from build123d import *

# Parameters (mm, degrees)
SKETCH1_R           = 18
SKETCH1_R_2         = 2
SKETCH1_W           = 10.25
SKETCH1_H           = 10.25
BOSS_EXTRUDE1_DEPTH = 36
CUT_EXTRUDE1_START  = -7
CUT_EXTRUDE1_DEPTH  = 7
SKETCH4_W           = 9.35
SKETCH4_H           = 9.35
CUT_EXTRUDE3_DEPTH  = 20.4
CUT_EXTRUDE4_START  = -40
CUT_EXTRUDE4_DEPTH  = 40
SKETCH6_R           = 1.5
CUT_EXTRUDE5_DEPTH  = 53.687759489
SKETCH7_R           = 3
CUT_EXTRUDE6_DEPTH  = 3
CUT_EXTRUDE7_DEPTH  = 4
CHAMFER1_SIZE       = 1
CHAMFER1_SIZE_2     = 2.747477419
CUT_EXTRUDE8_DEPTH  = 44.69210455
SKETCH12_R          = 1.4
CUT_EXTRUDE10_DEPTH = 20
SKETCH13_R          = 20
SKETCH13_R_2        = 1.4
BOSS_EXTRUDE2_DEPTH = 3
BOSS_EXTRUDE3_DEPTH = 3


with BuildPart() as part:
    # Sketch1 → Boss-Extrude1 (new body)
    with BuildSketch(Plane(origin=(0, 0, 0), x_dir=(1, 0, 0), z_dir=(0, 1, 0))):
        with Locations(Location((0, 0, 0), (0, 0, 270))):
            Circle(SKETCH1_R)
        with Locations(Location((-12, 0, 0), (0, 0, 270))):
            Circle(SKETCH1_R_2, mode=Mode.SUBTRACT)
        Rectangle(SKETCH1_W, SKETCH1_H, mode=Mode.SUBTRACT)
    extrude(amount=BOSS_EXTRUDE1_DEPTH)

    # Sketch2 → Cut-Extrude1 (cut)
    with BuildSketch(Plane(origin=(0, 36, 0), x_dir=(1, 0, 0), z_dir=(0, 1, 0)).offset(CUT_EXTRUDE1_START)):
        with BuildLine():
            Line((-10.8, 5), (-17.291616466, 5))
            ThreePointArc((-17.291616466, 5), (-18, 0), (-17.291616466, -5))
            Line((-17.291616466, -5), (-10.8, -5))
            ThreePointArc((-10.8, -5), (-5.8, 0), (-10.8, 5))
        make_face()
    extrude(amount=CUT_EXTRUDE1_DEPTH, mode=Mode.SUBTRACT)

    # Sketch4 → Cut-Extrude3 (cut)
    with BuildSketch(Plane(origin=(0, 0, 0), x_dir=(-1, 0, 0), z_dir=(0, -1, 0))):
        with Locations((11.135393506, 0.872889968)):
            Rectangle(SKETCH4_W, SKETCH4_H)
    extrude(amount=-CUT_EXTRUDE3_DEPTH, mode=Mode.SUBTRACT)

    # Sketch5 → Cut-Extrude4 (cut)
    with BuildSketch(Plane(origin=(0, 36, 0), x_dir=(1, 0, 0), z_dir=(0, 1, 0)).offset(CUT_EXTRUDE4_START)):
        with BuildLine():
            Line((5.916079783, 17), (-5.916079783, 17))
            ThreePointArc((-5.916079783, 17), (0, 18), (5.916079783, 17))
        make_face()
        with BuildLine():
            Line((5.916079783, -17), (-5.916079783, -17))
            ThreePointArc((-5.916079783, -17), (0, -18), (5.916079783, -17))
        make_face()
    extrude(amount=CUT_EXTRUDE4_DEPTH, mode=Mode.SUBTRACT)

    # Sketch6 → Cut-Extrude5 (cut, through all)
    with BuildSketch(Plane(origin=(0, 0, -17), x_dir=(-1, 0, 0), z_dir=(0, 0, -1))):
        with Locations((0, 26)):
            Circle(SKETCH6_R)
        with Locations((0, 5)):
            Circle(SKETCH6_R)
    extrude(amount=-CUT_EXTRUDE5_DEPTH, mode=Mode.SUBTRACT)

    # Sketch7 → Cut-Extrude6 (cut)
    with BuildSketch(Plane(origin=(0, 0, -17), x_dir=(-1, 0, 0), z_dir=(0, 0, -1))):
        with Locations((0, 26)):
            Circle(SKETCH7_R)
        with Locations((0, 5)):
            Circle(SKETCH7_R)
    extrude(amount=-CUT_EXTRUDE6_DEPTH, mode=Mode.SUBTRACT)

    # Sketch8 → Cut-Extrude7 (cut)
    with BuildSketch(Plane.XY.offset(17)):
        Polygon((0, 22.8), (2.771281292, 24.4), (2.771281292, 27.6), (0, 29.2), (-2.771281292, 27.6), (-2.771281292, 24.4), align=None)
        Polygon((0, 1.8), (2.771281292, 3.4), (2.771281292, 6.6), (0, 8.2), (-2.771281292, 6.6), (-2.771281292, 3.4), align=None)
    extrude(amount=-CUT_EXTRUDE7_DEPTH, mode=Mode.SUBTRACT)

    # Chamfer1
    # the kernel refuses this chamfer: 2.747477419, 1 mm, written as the material it takes off along each edge
    with BuildSketch(Plane(origin=(-5.125, 36, -5.125), x_dir=(0, 0.09904090225204956, -0.9950833631817488), z_dir=(1, 0, 0)), Plane(origin=(-5.125, 36, 5.125), x_dir=(-0.9950833631817488, 0.09904090225204956, 0), z_dir=(0, 0, -1)), Plane(origin=(5.125, 36, 5.125), x_dir=(0, 0.09904090225204956, 0.9950833631817488), z_dir=(-1, 0, 0)), Plane(origin=(5.125, 36, -5.125), x_dir=(0.9950833631817488, 0.09904090225204956, 0), z_dir=(0, 0, 1))) as chamfer1_piece_1:
        Polygon((CHAMFER1_SIZE * 0.995083363182, -CHAMFER1_SIZE * 0.099040902252), (-CHAMFER1_SIZE_2 * 0.0990409022684, -CHAMFER1_SIZE_2 * 0.995083363346), (0, 0), align=None)
    extrude(amount=10.25, mode=Mode.SUBTRACT)
    with BuildSketch(Plane(origin=(-5.125, 36, 5.125), x_dir=(-0.9950833631817488, 0.09904090225204956, 0), z_dir=(0, 0, -1))) as chamfer1_piece_2a_section:
        Polygon((CHAMFER1_SIZE * 0.995083363182, -CHAMFER1_SIZE * 0.099040902252), (-CHAMFER1_SIZE_2 * 0.0990409022684, -CHAMFER1_SIZE_2 * 0.995083363346), (0, 0), align=None)
    chamfer1_piece_2a = extrude(amount=17.377491449, mode=Mode.PRIVATE)
    chamfer1_piece_2a = split(chamfer1_piece_2a, bisect_by=Plane(origin=(-5.432505006, 35.059901151, -5.125), z_dir=(0, 0, -1)), keep=Keep.TOP, mode=Mode.PRIVATE)
    with BuildSketch(Plane(origin=(-12.252491449, 36, -5.125), x_dir=(0, 0.09904090225204956, -0.9950833631817488), z_dir=(1, 0, 0))) as chamfer1_piece_2b_section:
        Polygon((CHAMFER1_SIZE * 0.995083363182, -CHAMFER1_SIZE * 0.099040902252), (-CHAMFER1_SIZE_2 * 0.0990409022684, -CHAMFER1_SIZE_2 * 0.995083363346), (0, 0), align=None)
    chamfer1_piece_2b = extrude(amount=17.377491449, mode=Mode.PRIVATE)
    chamfer1_piece_2b = split(chamfer1_piece_2b, bisect_by=Plane(origin=(-5.125, 35.059901151, -5.432505006), z_dir=(-1, 0, 0)), keep=Keep.TOP, mode=Mode.PRIVATE)
    chamfer1_piece_2 = chamfer1_piece_2a & chamfer1_piece_2b
    add(chamfer1_piece_2, mode=Mode.SUBTRACT)
    with BuildSketch(Plane(origin=(5.125, 36, -12.252491449), x_dir=(0.9950833631817488, 0.09904090225204956, 0), z_dir=(0, 0, 1))) as chamfer1_piece_3a_section:
        Polygon((CHAMFER1_SIZE * 0.995083363182, -CHAMFER1_SIZE * 0.099040902252), (-CHAMFER1_SIZE_2 * 0.0990409022684, -CHAMFER1_SIZE_2 * 0.995083363346), (0, 0), align=None)
    chamfer1_piece_3a = extrude(amount=17.377491449, mode=Mode.PRIVATE)
    chamfer1_piece_3a = split(chamfer1_piece_3a, bisect_by=Plane(origin=(5.432505006, 35.059901151, -5.125), z_dir=(0, 0, -1)), keep=Keep.TOP, mode=Mode.PRIVATE)
    with BuildSketch(Plane(origin=(-5.125, 36, -5.125), x_dir=(0, 0.09904090225204956, -0.9950833631817488), z_dir=(1, 0, 0))) as chamfer1_piece_3b_section:
        Polygon((CHAMFER1_SIZE * 0.995083363182, -CHAMFER1_SIZE * 0.099040902252), (-CHAMFER1_SIZE_2 * 0.0990409022684, -CHAMFER1_SIZE_2 * 0.995083363346), (0, 0), align=None)
    chamfer1_piece_3b = extrude(amount=17.377491449, mode=Mode.PRIVATE)
    chamfer1_piece_3b = split(chamfer1_piece_3b, bisect_by=Plane(origin=(5.125, 35.059901151, -5.432505006), z_dir=(1, 0, 0)), keep=Keep.TOP, mode=Mode.PRIVATE)
    chamfer1_piece_3 = chamfer1_piece_3a & chamfer1_piece_3b
    add(chamfer1_piece_3, mode=Mode.SUBTRACT)
    with BuildSketch(Plane(origin=(5.125, 36, 5.125), x_dir=(0, 0.09904090225204956, 0.9950833631817488), z_dir=(-1, 0, 0))) as chamfer1_piece_4a_section:
        Polygon((CHAMFER1_SIZE * 0.995083363182, -CHAMFER1_SIZE * 0.099040902252), (-CHAMFER1_SIZE_2 * 0.0990409022684, -CHAMFER1_SIZE_2 * 0.995083363346), (0, 0), align=None)
    chamfer1_piece_4a = extrude(amount=17.377491449, mode=Mode.PRIVATE)
    chamfer1_piece_4a = split(chamfer1_piece_4a, bisect_by=Plane(origin=(-5.125, 35.059901151, 5.432505006), z_dir=(-1, 0, 0)), keep=Keep.TOP, mode=Mode.PRIVATE)
    with BuildSketch(Plane(origin=(-5.125, 36, 12.252491449), x_dir=(-0.9950833631817488, 0.09904090225204956, 0), z_dir=(0, 0, -1))) as chamfer1_piece_4b_section:
        Polygon((CHAMFER1_SIZE * 0.995083363182, -CHAMFER1_SIZE * 0.099040902252), (-CHAMFER1_SIZE_2 * 0.0990409022684, -CHAMFER1_SIZE_2 * 0.995083363346), (0, 0), align=None)
    chamfer1_piece_4b = extrude(amount=17.377491449, mode=Mode.PRIVATE)
    chamfer1_piece_4b = split(chamfer1_piece_4b, bisect_by=Plane(origin=(-5.432505006, 35.059901151, 5.125), z_dir=(0, 0, 1)), keep=Keep.TOP, mode=Mode.PRIVATE)
    chamfer1_piece_4 = chamfer1_piece_4a & chamfer1_piece_4b
    add(chamfer1_piece_4, mode=Mode.SUBTRACT)
    with BuildSketch(Plane(origin=(12.252491449, 36, 5.125), x_dir=(0, 0.09904090225204956, 0.9950833631817488), z_dir=(-1, 0, 0))) as chamfer1_piece_5a_section:
        Polygon((CHAMFER1_SIZE * 0.995083363182, -CHAMFER1_SIZE * 0.099040902252), (-CHAMFER1_SIZE_2 * 0.0990409022684, -CHAMFER1_SIZE_2 * 0.995083363346), (0, 0), align=None)
    chamfer1_piece_5a = extrude(amount=17.377491449, mode=Mode.PRIVATE)
    chamfer1_piece_5a = split(chamfer1_piece_5a, bisect_by=Plane(origin=(5.125, 35.059901151, 5.432505006), z_dir=(1, 0, 0)), keep=Keep.TOP, mode=Mode.PRIVATE)
    with BuildSketch(Plane(origin=(5.125, 36, -5.125), x_dir=(0.9950833631817488, 0.09904090225204956, 0), z_dir=(0, 0, 1))) as chamfer1_piece_5b_section:
        Polygon((CHAMFER1_SIZE * 0.995083363182, -CHAMFER1_SIZE * 0.099040902252), (-CHAMFER1_SIZE_2 * 0.0990409022684, -CHAMFER1_SIZE_2 * 0.995083363346), (0, 0), align=None)
    chamfer1_piece_5b = extrude(amount=17.377491449, mode=Mode.PRIVATE)
    chamfer1_piece_5b = split(chamfer1_piece_5b, bisect_by=Plane(origin=(5.432505006, 35.059901151, 5.125), z_dir=(0, 0, 1)), keep=Keep.TOP, mode=Mode.PRIVATE)
    chamfer1_piece_5 = chamfer1_piece_5a & chamfer1_piece_5b
    add(chamfer1_piece_5, mode=Mode.SUBTRACT)

    # Sketch9 → Cut-Extrude8 (cut, through all)
    with BuildSketch(Plane.XZ):
        with BuildLine():
            Line((-7.454203172, -7.297889968), (-15.454203172, -7.297889968))
            ThreePointArc((-15.454203172, -7.297889968), (-13.761984914, -9.955415688), (-11.632322635, -12.277178848))
            Line((-11.632322635, -12.277178848), (-7.454203172, -7.297889968))
        make_face()
    extrude(amount=-CUT_EXTRUDE8_DEPTH, mode=Mode.SUBTRACT)

    # Sketch12 → Cut-Extrude10 (cut)
    with BuildSketch(Plane(origin=(0, 36, 0), x_dir=(1, 0, 0), z_dir=(0, 1, 0))):
        with Locations(Location((10, 0, 0), (0, 0, 270))):
            Circle(SKETCH12_R)
        with Locations(Location((-9.192388155, -9.192388155, 0), (0, 0, 270))):
            Circle(SKETCH12_R)
    extrude(amount=-CUT_EXTRUDE10_DEPTH, mode=Mode.SUBTRACT)

    # Sketch13 → Boss-Extrude2 (add)
    with BuildSketch(Plane(origin=(0, 36, 0), x_dir=(1, 0, 0), z_dir=(0, 1, 0))):
        with Locations(Location((0, 0, 0), (0, 0, 270))):
            Circle(SKETCH13_R)
        with Locations(Location((10, 0, 0), (0, 0, 270))):
            Circle(SKETCH13_R_2, mode=Mode.SUBTRACT)
        with Locations(Location((-9.192388155, -9.192388155, 0), (0, 0, 270))):
            Circle(SKETCH13_R_2, mode=Mode.SUBTRACT)
        with BuildLine():
            Line((-10.8, 5), (-17.291616466, 5))
            Line((-17.291616466, 5), (-17.291616466, -5))
            Line((-17.291616466, -5), (-10.8, -5))
            ThreePointArc((-10.8, -5), (-7.959770503, -4.114984375), (-6.125, -1.773238563))
            Line((-6.125, -1.773238563), (-6.125, -6.125))
            Line((-6.125, -6.125), (6.125, -6.125))
            Line((6.125, -6.125), (6.125, 6.125))
            Line((6.125, 6.125), (-6.125, 6.125))
            Line((-6.125, 6.125), (-6.125, 1.773238563))
            ThreePointArc((-6.125, 1.773238563), (-7.959770503, 4.114984375), (-10.8, 5))
        make_face(mode=Mode.SUBTRACT)
        with BuildLine():
            Line((-7.454203172, 7.297889968), (-15.454203172, 7.297889968))
            ThreePointArc((-15.454203172, 7.297889968), (-13.761984914, 9.955415688), (-11.632322635, 12.277178848))
            Line((-11.632322635, 12.277178848), (-7.454203172, 7.297889968))
        make_face(mode=Mode.SUBTRACT)
    extrude(amount=BOSS_EXTRUDE2_DEPTH)

    # Sketch14 → Boss-Extrude3 (add)
    with BuildSketch(Plane(origin=(0, 39, 0), x_dir=(1, 0, 0), z_dir=(0, 1, 0))):
        with BuildLine():
            Line((12.855752194, 15.320888862), (14.321646009, 13.960317173))
            ThreePointArc((14.321646009, 13.960317173), (14.268984946, 15.373549926), (12.855752194, 15.320888862))
        make_face()
    extrude(amount=-BOSS_EXTRUDE3_DEPTH)


solid = part.part
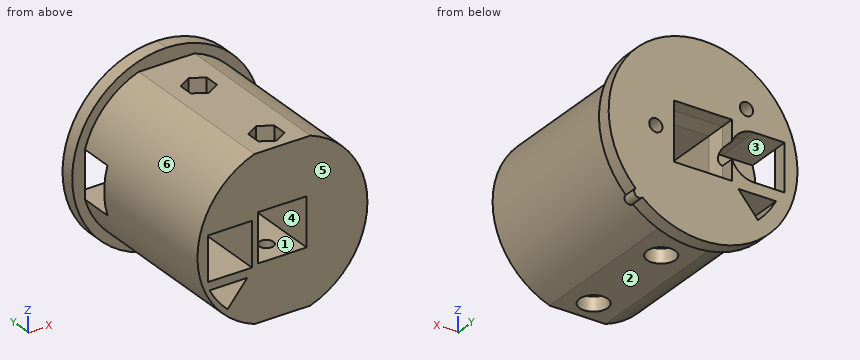
CAD build for the part. Positions are in the model's coordinates, mm. Face numbers are marked on the shaded views. A direction names the side the tool comes from. Coordinates: 2 decimals unless noted, no trailing zeros. Write each loop counter-clockwise with the first axis right and the second up, starting at its lowest first coordinate (ties: lowest second). Pieces come first, ordered by that corner, then holes. Notation, with made-up numbers: M 72.5,85.25 L 91.5,85.25 A12 ccw 91.5,96.25 Z; hole C 11.25,28.5 d7. An arc over 180 degrees is marked long. Answer as a JSON object with one key per item and string values. Group by question number.
1) Saw through at C-C (y = 19). Write the cut outline in (x, z) (3 decimals).
2) Saw through at D-D (z = -4). Write the cut outline in (x, y) (3 decimals), plus the area to 3 significant figures.
3) Mould opens along Z. For the marked faces 4, 5 and 6 say: +Z half, -Z half, draft (parallel to the pull), parting line (faces both ways), or undercut.
4) Saw through at A-A (y = 26). Give the number of separate pieces and of enclosed holes in the cut face, plus the area to 3 significant figures.
5) Saw through at B-B (z = -9.5). Write the cut outline in (x, y), plus the area to 3 significant figures.
6) Wall check: line 1 (X direction, y = 24.5, z = 0) (3 decimals); line 2 (Y direction, x = 0, z = -15); line 3 (Y direction, x = 0, z = -9). Give the ranges that are in metal, low to high. Write a range as from..to.
7) Pin check, flat tips, straight feed: pin 1 Ø5 at (x, y) = (-15, 32) entering from -Z; pin 2 Ø1.5 at (y, z) = (21, 14) entering from -X; pin 3 Ø8 at (y, z) = (14.5, -1) entering from +X. Stop position of each tip, or through.
8) Tool access for the marked faces 1, 2 and 3: list every direction of +Z, -Z, +X, -X, +Y, -Y with a clear straight run to the whole face (end or side of a thin tool).
Values follow:
{
 "1": {"outline": "M -5.916,-17 L 5.916,-17 A18 ccw 5.916,17 L -5.916,17 A18 ccw Z; hole M -15.81,-5.548 L -6.46,-5.548 L -6.46,3.802 L -15.81,3.802 Z; hole M -15.454,-7.298 A18 ccw -11.632,-12.277 L -7.454,-7.298 Z; hole C -9.192,9.192 d2.8; hole M -5.125,-5.125 L 5.125,-5.125 L 5.125,5.125 L -5.125,5.125 Z; hole C 10,0 d2.8"},
 "2": {"outline": "M -19.596,36 L -17.292,36 L -17.292,39 L -19.596,39 Z; M -17.55,0 L -15.81,0 L -15.81,20.4 L -6.46,20.4 L -6.46,0 L -5.125,0 L -5.125,33.253 L -6.125,36 L -6.125,39 L -7.8,39 L -7.8,29 L -17.55,29 Z; M 5.125,0 L 17.55,0 L 17.55,36 L 19.596,36 L 19.596,39 L 6.125,39 L 6.125,36 L 5.125,33.253 Z", "area": "685 mm2"},
 "3": {"face 4": "undercut", "face 5": "draft", "face 6": "parting line"},
 "4": {"separate pieces": "2", "enclosed holes": "4", "area": "761 mm2"},
 "5": {"outline": "M -17.6,36 L -15.29,36 L -15.29,0 L -14.1,0 L -14.1,39 L -17.6,39 Z; M -9.3,0 L 15.29,0 L 15.29,36 L 17.6,36 L 17.6,39 L -9.3,39 Z; hole C 0,5 d3; hole C 0,26 d3", "area": "1,010 mm2"},
 "6": {"line 1": "x = -18..-14, -10..-5.125, 5.125..8.6, 11.4..18", "line 2": "y = 0..2, 8..23, 29..39", "line 3": "y = 0..3.5, 6.5..24.5, 27.5..39"},
 "7": {"pin 1": "stops at z = -12.95", "pin 2": "stops at x = -12.18", "pin 3": "stops at x = 18"},
 "8": {"face 1": "+Y, -Y", "face 2": "-Z, +X, -X, -Y", "face 3": "+Y"}
}
